Geometry check sheet. Reference: the model listing, model coordinates, mm. Face numbers are marked on the shaded views. A direction names the side the tool comes from. Coordinates: 2 decimals unless noted, no trailing zeros. Order: outer loops, then holes, each group sorted by start corner. A loop starts at its lowest first (then second) coordinate and runs counter-clockwise, first axis right, second up. Notation, with made-up numbers: (71, -28) - (112, -28) arc R32 ccw to (112, -1) - close; hole circle Ø8 at (10, 87.25). An arc over 180 degrees is marked (long way). Put each result on its own line as item: value.
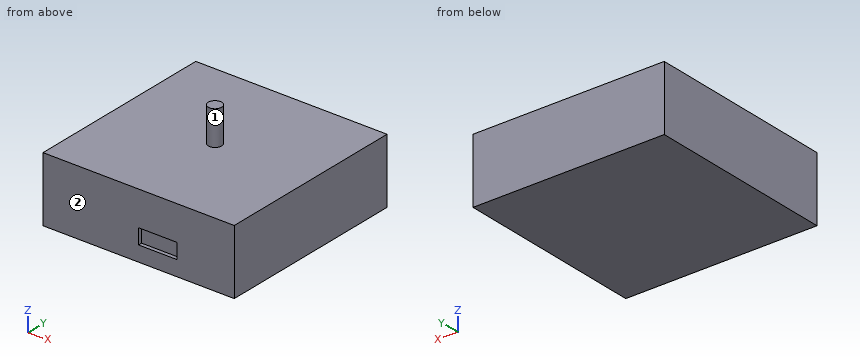
from build123d import *

# Parameters (mm, degrees)
SKETCH_W     = 50
SKETCH_H     = 50
PAD_DEPTH    = 17
SKETCH001_R  = 1.75
PAD001_DEPTH = 9
SKETCH002_W  = 10
SKETCH002_H  = 4
POCKET_DEPTH = 1


with BuildPart() as part:
    # Sketch → Pad (new body)
    with BuildSketch(Plane.XY):
        Rectangle(SKETCH_W, SKETCH_H)
    extrude(amount=PAD_DEPTH)

    # Sketch001 (on Face6 of Pad) → Pad001 (join)
    with BuildSketch(Plane.XY.offset(17)):
        Circle(SKETCH001_R)
    extrude(amount=PAD001_DEPTH)

    # Sketch002 (on Face6 of Pad001) → Pocket (cut)
    with BuildSketch(Plane.XZ.offset(25)):
        with Locations((5, 6)):
            Rectangle(SKETCH002_W, SKETCH002_H)
    extrude(amount=-POCKET_DEPTH, mode=Mode.SUBTRACT)


solid = part.part
Q1. Section check B-B on x = 22. Record the boundary of the cut face in (y, z), then the cut area to 3 significant figures.
Answer block:
outline: (-25, 0) - (25, 0) - (25, 17) - (-25, 17) - close
area: 850 mm^2
Q2. Section check A-A on y = 0. Record the boundary of the cut face in (x, z), then the cut area to 4 significant figures.
Answer block:
outline: (-25, 0) - (25, 0) - (25, 17) - (1.75, 17) - (1.75, 26) - (-1.75, 26) - (-1.75, 17) - (-25, 17) - close
area: 881.5 mm^2
Q3. Depth check by flat-ended pin: pin 1 Ø12 at (x, y) = (13, -14.5) entering from +Z. Enter the tip coordinate at first touch or a pass-through.
Answer block:
pin 1: stops at z = 17
Q4. Thickness scan on L1, parallel to Z at x = 8.5, y = 12.5; L2, parallel to Y at x = 7.5, z = 5.75. Record the ranges inside material, lowest first. Write a range as [from, to].
Answer block:
L1: z = [0, 17]
L2: y = [-24, 25]
Q5. Access from +Z, -Z, +X, -X, +Y, -Y to the whole of each face (thin tool, end or side, straight path). Record for the marked faces 1 and 2.
Answer block:
face 1: +Z
face 2: +Z, -Z, +X, -X, -Y
